Geometry: final body of the model. Coordinates: model frame, mm. A direction names the side the tool comes from. Round coordinates to 2 decimals unless told otherwise and drop trailing zeros. Loops run counter-clockwise (first coordinate to the right, second up) from the corner with the lowest first, then second, coordinate; pieces in that order, holes last. Notation, with made-up numbers: (31.5, -34.75) - (63.5, -34.75) arc R19 cw to (63.5, -25.75) - close; hole circle Ø8 at (8.5, 84.5). An arc over 180 degrees is marked (long way). Use CSV: the item, a comma, the result in double quotes.
from build123d import *

# Parameters (mm, degrees)
F0_R     = 7.35
F1_DEPTH = 5.842
F2_R     = 2
F3_W     = 3.0988
F3_H     = 6.35
F4_DEPTH = 25.4
F5_W     = 12.7
F5_H     = 3.0988
F6_DEPTH = 5.842
F8_DEPTH = 5.842


with BuildPart() as f1:
    # F0 (on Front) → F1 (new body)
    with BuildSketch(Plane.XZ):
        Polygon((31.75, 11.1125), (-31.75, 11.1125), (-31.75, -11.1125), (-11.43, -11.1125), (-7.62, -1.5875), (0, -1.5875), (7.62, -1.5875), (11.43, -11.1125), (31.75, -11.1125), align=None)
        with Locations((-19.05, 0)):
            Circle(F0_R, mode=Mode.SUBTRACT)
        with Locations((19.05, 0)):
            Circle(F0_R, mode=Mode.SUBTRACT)
    extrude(amount=F1_DEPTH)

    # F2
    f2_edges = [f1.edges().sort_by_distance(p)[0] for p in [
        (-11.43, -2.921, -11.1125),
        (-7.62, -2.921, -1.5875),
        (7.62, -2.921, -1.5875),
        (11.43, -2.921, -11.1125),
    ]]
    fillet(f2_edges, radius=F2_R)

    # F3 (on face) → F4 (cut)
    with BuildSketch(Plane(origin=(0, 0, 0), x_dir=(-1, 0, 0), z_dir=(0, 1, 0))):
        with Locations((4.7625, 4.7625)):
            Rectangle(F3_W, F3_H)
    extrude(amount=-F4_DEPTH, mode=Mode.SUBTRACT)

    # F5 (on face) → F6 (join, through all)
    with BuildSketch(Plane.XZ.offset(5.842)):
        with Locations((-12.7, 12.6619)):
            Rectangle(F5_W, F5_H)
        with Locations((12.7, 12.6619)):
            Rectangle(F5_W, F5_H)
    extrude(amount=-F6_DEPTH)

    # F7 (on face) → F8 (join, through all)
    with BuildSketch(Plane.XZ.offset(5.842)):
        Polygon((38.592, 6.35), (32.75, 6.35), (32.75, 11.1125), (31.75, 11.1125), (31.75, 6.35), (31.75, -6.35), (31.75, -11.1125), (32.75, -11.1125), (32.75, -6.35), (38.592, -6.35), align=None)
        Polygon((-31.75, 6.35), (-31.75, 11.1125), (-32.75, 11.1125), (-32.75, 6.35), (-38.592, 6.35), (-38.592, -6.35), (-32.75, -6.35), (-32.75, -11.1125), (-31.75, -11.1125), (-31.75, -6.35), align=None)
    extrude(amount=-F8_DEPTH)


solid = f1.part
Item 1: Mould query, pull axis X, two halves, no side actions, for faces 4 (the flat face through (32.75, -3, 9)), 5 (the flat face through (0, -3, -1.588)), 6 (the flat face through (26, -3, 11.112)). Classes: released by +X, released by -X, zero draft, split by the parting line, or undercut.
Final values:
face 4,"released by +X"
face 5,"undercut"
face 6,"zero draft"
Item 2: Section A-A on y = -3.2. Give the number of separate pieces and of enclosed holes in the cut face, plus the area to 3 significant figures.
Final values:
separate pieces,"1"
enclosed holes,"3"
area,"1,140 mm²"
Item 3: Pin query (flat end, axial travel): P1, Ø3, axis at x = 34.5, y = -2, coming from the +Z side; P2, Ø0.9, axis at x = -4.5, y = -2.5, coming from the -Z side; P3, Ø1.4, axis at y = -4, z = 8, coming from the -X side. Return the tip coordinate at first contact, or that it passes through.
Final values:
P1,"stops at z = 6.35"
P2,"stops at z = -1.59"
P3,"stops at x = -32.75"
Item 4: Section C-C on z = 4. Return the cut outline in (x, y).
Final values:
outline,"(-38.59, -5.84) - (-25.22, -5.84) - (-25.22, 0) - (-38.59, 0) - close; (-12.88, -5.84) - (-6.31, -5.84) - (-6.31, 0) - (-12.88, 0) - close; (-3.21, -5.84) - (12.88, -5.84) - (12.88, 0) - (-3.21, 0) - close; (25.22, -5.84) - (38.59, -5.84) - (38.59, 0) - (25.22, 0) - close"
Item 5: Reachability of faces 1 (the cylindrical face through (7.4, -2.96, -1.94)), 2 (the flat face through (-6.35, -3, 13)), 3 (the flat face through (-36, -3, -6.35)) from +Z, -Z, +X, -X, +Y, -Y: full face, straight path, thin tool, end or side. Return the list, or none.
Final values:
face 1,"-Z, +Y, -Y"
face 2,"+Z, +Y, -Y"
face 3,"-Z, -X, +Y, -Y"
Item 6: Material intervals for line 1 (X direction, y = -3.35, z = 1.75); line 2 (X direction, y = -1.4, z = 6.5); line 3 (X direction, y = -1.3, z = 9.5), sorted ascending.
Final values:
line 1,"x = -38.59 to -26.19, -11.91 to -6.31, -3.21 to 11.91, 26.19 to 38.59"
line 2,"x = -32.75 to -22.48, -15.62 to -6.31, -3.21 to 15.62, 22.48 to 32.75"
line 3,"x = -32.75 to 32.75"
Item 7: Section B-B on z = 0.75. Return the cut outline in (x, y), plus the area to 3 significant figures.
Final values:
outline,"(-38.59, -5.84) - (-26.36, -5.84) - (-26.36, 0) - (-38.59, 0) - close; (-11.74, -5.84) - (11.74, -5.84) - (11.74, 0) - (-11.74, 0) - close; (26.36, -5.84) - (38.59, -5.84) - (38.59, 0) - (26.36, 0) - close"
area,"280 mm²"
Item 8: Section D-D on x = 32. Return the cut outline in (y, z).
Final values:
outline,"(-5.84, -11.11) - (0, -11.11) - (0, 11.11) - (-5.84, 11.11) - close"
